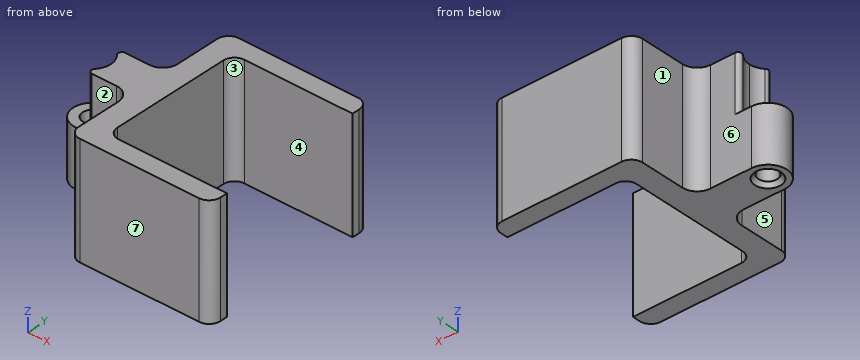
from build123d import *

# Parameters (mm, degrees)
F1_DEPTH    = 30
F2_DEPTH    = 30
F3_DEPTH    = 15
F4_R        = 2.5
F5_DEPTH    = 25
F6_R        = 3
F7_R        = 4
F8_T1_DEPTH = 26.1803398875
F9_SIZE     = 1


# Not quite as in the source:
# - a fillet or chamfer that OpenCascade refuses, or shapes differently, is made with other operations: its cross-section is extruded or revolved along the edge and cut away or added


with BuildPart() as f1:
    # F0 (on Top) → F1 (new body)
    with BuildSketch(Plane.XY):
        with BuildLine():
            ThreePointArc((-71.5824067593, 19.101677686), (-68.0468728533, 17.6372115919), (-66.5824067593, 14.101677686))
            ThreePointArc((-66.5824067593, 14.101677686), (-68.0468728533, 10.56614378), (-71.5824067593, 9.101677686))
            Line((-71.5824067593, 9.101677686), (-56.5824067593, 9.101677686))
            Line((-56.5824067593, 9.101677686), (-56.5824067593, 19.101677686))
            Line((-56.5824067593, 19.101677686), (-71.5824067593, 19.101677686))
        make_face()
    extrude(amount=F1_DEPTH)

    # F0 (on Top) → F2 (join)
    with BuildSketch(Plane.XY):
        Polygon((-56.5824067593, 38.101677686), (-56.5824067593, 33.101677686), (-50.5824067593, 33.101677686), (-18.5824067593, 33.101677686), (-18.5824067593, 38.101677686), align=None)
        Polygon((-56.5824067593, 33.101677686), (-56.5824067593, 19.101677686), (-56.5824067593, 9.101677686), (-56.5824067593, -4.898322314), (-50.5824067593, -4.898322314), (-50.5824067593, 33.101677686), align=None)
        Polygon((-50.5824067593, -4.898322314), (-56.5824067593, -4.898322314), (-56.5824067593, -9.898322314), (-18.5824067593, -9.898322314), (-18.5824067593, -4.898322314), align=None)
    extrude(amount=F2_DEPTH)

    # F0 (on Top) → F3 (join)
    with BuildSketch(Plane.XY):
        with BuildLine():
            ThreePointArc((-71.5824067593, 9.101677686), (-68.0468728533, 10.56614378), (-66.5824067593, 14.101677686))
            ThreePointArc((-66.5824067593, 14.101677686), (-68.0468728533, 17.6372115919), (-71.5824067593, 19.101677686))
            Line((-71.5824067593, 19.101677686), (-71.5824067593, 9.101677686))
        make_face()
        with BuildLine():
            Line((-71.5824067593, 9.101677686), (-71.5824067593, 19.101677686))
            ThreePointArc((-71.5824067593, 19.101677686), (-76.5824067593, 14.101677686), (-71.5824067593, 9.101677686))
        make_face()
    extrude(amount=F3_DEPTH)

    # F4 (on face) → F5 (cut)
    with BuildSketch(Plane.XY.offset(15)):
        with Locations((-71.5824067593, 14.101677686)):
            Circle(F4_R)
    extrude(amount=-F5_DEPTH, mode=Mode.SUBTRACT)

    # F6
    f6_edges = [f1.edges().sort_by_distance(p)[0] for p in [
        (-18.582407, -9.898322, 15),
        (-18.582407, 38.101678, 15),
        (-50.582407, 33.101678, 15),
        (-50.582407, -4.898322, 15),
        (-56.582407, -9.898322, 15),
        (-56.582407, 38.101678, 15),
    ]]
    fillet(f6_edges, radius=F6_R)

    # F7
    f7_edges = [f1.edges().sort_by_distance(p)[0] for p in [
        (-56.582407, 9.101678, 15),
        (-56.582407, 19.101678, 15),
    ]]
    fillet(f7_edges, radius=F7_R)

    # F8: fillet of radius 1 on 4 edges, made by hand

    # F8_s2 → F8_t1 (cut)
    with BuildSketch(Plane.XY.offset(15)):
        with BuildLine():
            ThreePointArc((-67.1102708043, 19.101677686), (-68.0231417334, 18.5099259764), (-67.8556267968, 17.4350110193))
            ThreePointArc((-67.8556267968, 17.4350110193), (-69.5411653069, 18.6660323319), (-71.5824067593, 19.101677686))
            Line((-71.5824067593, 19.101677686), (-67.1102708043, 19.101677686))
        make_face()
        with BuildLine():
            ThreePointArc((-67.1102708043, 9.101677686), (-68.0231417334, 9.6934293955), (-67.8556267968, 10.7683443526))
            ThreePointArc((-67.8556267968, 10.7683443526), (-69.5411653069, 9.5373230401), (-71.5824067593, 9.101677686))
            Line((-71.5824067593, 9.101677686), (-67.1102708043, 9.101677686))
        make_face()
    extrude(amount=F8_T1_DEPTH, mode=Mode.SUBTRACT)

    # F9
    f9_edges = [f1.edges().sort_by_distance(p)[0] for p in [
        (-74.082407, 14.101678, 0),
    ]]
    chamfer(f9_edges, length=F9_SIZE)


solid = f1.part
Here's how the part is built. I have some questions about the finished solid (model axes, mm). Face numbers are marked on the shaded views. A direction names the side the tool comes from. Give positions to 0.01 mm unless a question says otherwise; leave off trailing zeros. Order: outer loops, then holes, each group sorted by start corner. A loop starts at its lowest first (then second) coordinate and runs counter-clockwise, first axis right, second up. Notation, with made-up numbers: (-36.5, -13.75) -> (-23.5, -13.75) arc R26 ccw to (-23.5, 1.25) -> close; hole circle Ø10 at (63, -3.5). An arc over 180 degrees is marked (long way). Use a Markdown table: item, result. Add a question column.
Item 1: Imagine slicing it at D-D on y = 28.5. Please give me the cut outline in (x, z).
Item 2: Imagine slicing it at C-C on z = 23.75. Please give me the cut outline in (x, y), plus the area to 3 significant figures.
Item 3: Imagine slicing it at A-A on z = 9.5. Please give me the cut outline in (x, y), plus the area to 3 significant figures.
Item 4: Will these pins go through, and if not, where does the flat tip stop? pin 1 (1.5 mm diameter, centred on x = -60, y = 6.5, fed in from -Z); pin 2 (9.5 mm diameter, centred on y = 26.5, z = 12, fed in from -X); pin 3 (6 mm diameter, centred on y = -1, z = 19.5, fed in from -X); pin 4 (4 mm diameter, centred on x = -56, z = 18, fed in from +Y).
Item 5: For the marked faces 1, 2 and 3, which set-ups out of +Z, -Z, +X, -X, +Y, -Y let a thin tool reach every point of the face, with its end or its side?
Item 6: If we mould it in two halves opening along Y, with no side actions, what happens to the marked faces 4, 5, 6 and 7? For each: pulls with the +Y half, pulls with the -Y half, needs draft (parallel to the pull), parting line crosses it, or undercut.
Item 7: Imagine slicing it at B-B on x = -25. Please give me the cut outline in (y, z), plus the area to 3 significant figures.
Item 8: I need wall thicknesses on line 1 (Y direction, x = -28.5, z = 26.25); line 2 (X direction, y = 18, z = 17.5); line 3 (X direction, y = 23.5, z = 26.25). Which ranges of each line are inside material? Lowest first, please.
Data:
| question | item | result |
|---|---|---|
| 1 | outline | (-56.58, 0) -> (-50.58, 0) -> (-50.58, 30) -> (-56.58, 30) -> close |
| 2 | outline | (-67.86, 10.77) arc R1 ccw to (-67.11, 9.1) -> (-60.58, 9.1) arc R4 cw to (-56.58, 5.1) -> (-56.58, -6.9) arc R3 ccw to (-53.58, -9.9) -> (-21.58, -9.9) arc R3 ccw to (-18.58, -6.9) -> (-18.58, -4.9) -> (-47.58, -4.9) arc R3 cw to (-50.58, -1.9) -> (-50.58, 30.1) arc R3 cw to (-47.58, 33.1) -> (-18.58, 33.1) -> (-18.58, 35.1) arc R3 ccw to (-21.58, 38.1) -> (-53.58, 38.1) arc R3 ccw to (-56.58, 35.1) -> (-56.58, 23.1) arc R4 cw to (-60.58, 19.1) -> (-67.11, 19.1) arc R1 ccw to (-67.86, 17.44) arc R5 cw to start |
| 2 | area | 718 mm² |
| 3 | outline | (-71.58, 9.1) -> (-60.58, 9.1) arc R4 cw to (-56.58, 5.1) -> (-56.58, -6.9) arc R3 ccw to (-53.58, -9.9) -> (-21.58, -9.9) arc R3 ccw to (-18.58, -6.9) -> (-18.58, -4.9) -> (-47.58, -4.9) arc R3 cw to (-50.58, -1.9) -> (-50.58, 30.1) arc R3 cw to (-47.58, 33.1) -> (-18.58, 33.1) -> (-18.58, 35.1) arc R3 ccw to (-21.58, 38.1) -> (-53.58, 38.1) arc R3 ccw to (-56.58, 35.1) -> (-56.58, 23.1) arc R4 cw to (-60.58, 19.1) -> (-71.58, 19.1) arc R5 ccw to start; hole circle Ø5 at (-71.58, 14.1) |
| 3 | area | 781 mm² |
| 4 | pin 1 | passes through |
| 4 | pin 2 | stops at x = -56.82 |
| 4 | pin 3 | stops at x = -56.58 |
| 4 | pin 4 | stops at y = 38.07 |
| 5 | face 1 | +Z, -Z, -X, +Y |
| 5 | face 2 | +Z, -Z, -X, -Y |
| 5 | face 3 | +Z, -Z, +X |
| 6 | face 4 | undercut |
| 6 | face 5 | needs draft |
| 6 | face 6 | pulls with the +Y half |
| 6 | face 7 | pulls with the -Y half |
| 7 | outline | (-9.9, 0) -> (-4.9, 0) -> (-4.9, 30) -> (-9.9, 30) -> close; (33.1, 0) -> (38.1, 0) -> (38.1, 30) -> (33.1, 30) -> close |
| 7 | area | 300 mm² |
| 8 | line 1 | y = -9.9 to -4.9, 33.1 to 38.1 |
| 8 | line 2 | x = -68.11 to -50.58 |
| 8 | line 3 | x = -56.58 to -50.58 |
